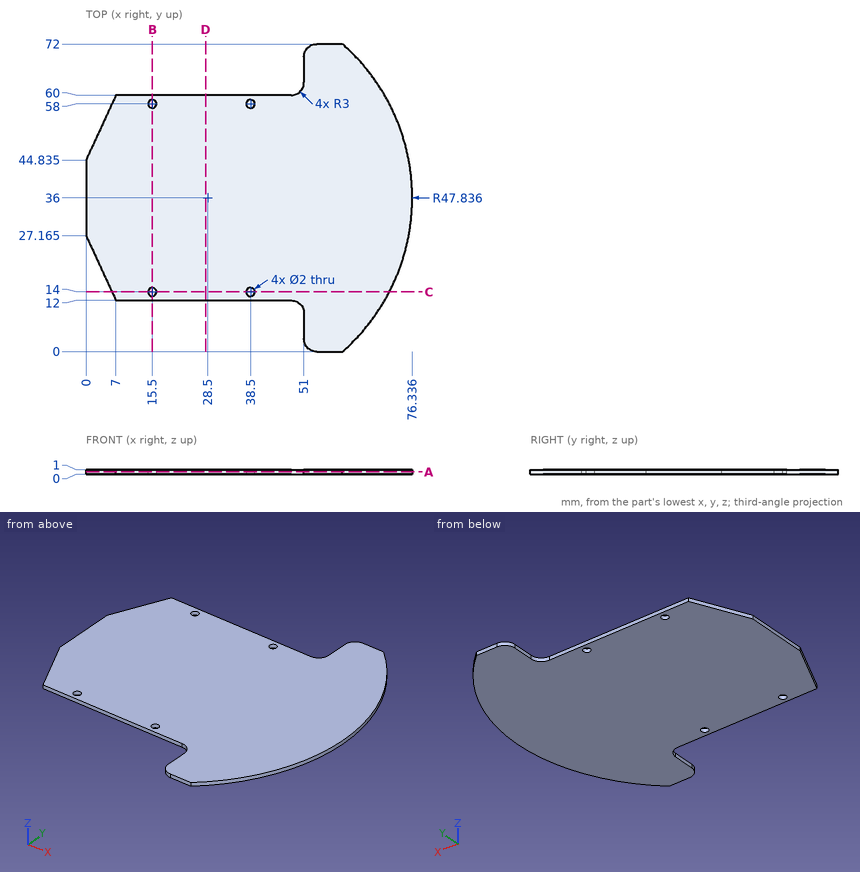
Here's the drawing with two shaded views (mm, measured from the low corner). I have some questions. Coordinates: 2 decimals unless noted, no trailing zeros. Write each loop counter-clockwise with the first axis right and the second up, starting at its lowest first coordinate (ties: lowest second). Pieces come first, ordered by that corner, then holes. Notation, with made-up numbers: M 89.25,-22 L 99.25,-22 A27 ccw 99.25,-4 Z; hole C 79,83 d5. An arc over 180 degrees is marked long. Answer as CSV lines item,"result". Start each with the question number.
1) I want a section at B-B, the plane x = 15.5. Please give me the cut outline in (y, z).
2) I want a section at C-C, the plane y = 14. Please give me the cut outline in (x, z).
3) Please list where these lines run through material, in increasing order: line 1 (Y direction, x = 38.5, z = 0.4); line 2 (Y direction, x = 20, z = 0.65); line 3 (Y direction, x = 39, z = 0.4) (1 decimal). Write a range as from..to.
4) I want a section at A-A, the plane z = 0.5. Please give me the cut outline in (x, y) (1 decimal), and give its area (3 significant figures).
5) I want a section at D-D, the plane x = 28. Please give me the cut outline in (y, z).
Data:
1,outline,"M 12,0 L 13,0 L 13,1 L 12,1 Z; M 15,0 L 57,0 L 57,1 L 15,1 Z; M 59,0 L 60,0 L 60,1 L 59,1 Z"
2,outline,"M 6.08,0 L 14.5,0 L 14.5,1 L 6.08,1 Z; M 16.5,0 L 37.5,0 L 37.5,1 L 16.5,1 Z; M 39.5,0 L 70.98,0 L 70.98,1 L 39.5,1 Z"
3,line 1,"y = 12..13, 15..57, 59..60"
3,line 2,"y = 12..60"
3,line 3,"y = 12..13.1, 14.9..57.1, 58.9..60"
4,outline,"M 0,27.2 L 7,12 L 48,12 A3 cw 51,9 L 51,3 A3 ccw 54,0 L 60,0 A47.8 ccw 60,72 L 54,72 A3 ccw 51,69 L 51,63 A3 cw 48,60 L 7,60 L 0,44.8 Z; hole C 15.5,14 d2; hole C 15.5,58 d2; hole C 38.5,14 d2; hole C 38.5,58 d2"
4,area,"3,790 mm^2"
5,outline,"M 12,0 L 60,0 L 60,1 L 12,1 Z"
